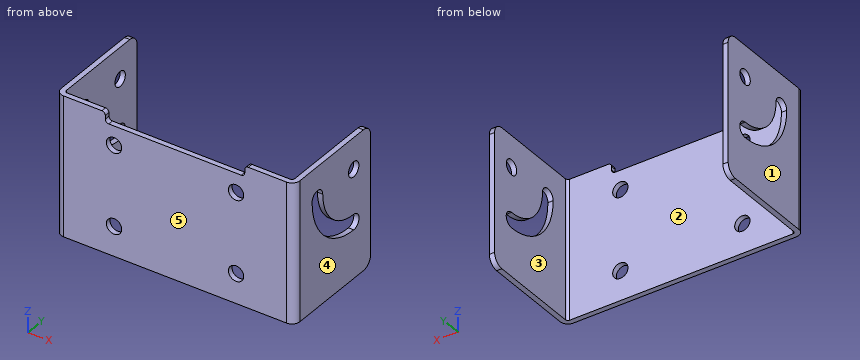
from build123d import *

# Parameters (mm, degrees)
SKETCH_1_W                         = 65.5
SKETCH_1_H                         = 40
SKETCH_1_R                         = 2.2
SM_BASE_FLANGE_1_DEPTH             = 1.5
SM_EDGE_FLANGE_1_STRIP_W           = 7.4732
SM_EDGE_FLANGE_1_STRIP_H           = 1.5
SM_EDGE_FLANGE_1_STRIP_CUT_DEPTH   = 40
SM_EDGE_FLANGE_1_STRIP_2_W         = 7.4732
SM_EDGE_FLANGE_1_STRIP_2_H         = 1.5
SM_EDGE_FLANGE_1_STRIP_CUT_2_DEPTH = 40
SM_EDGE_FLANGE_1_DEPTH             = 40
SM_EDGE_FLANGE_1_BEND_DEPTH        = 40
SKETCH_12_R                        = 2.15
CUT_EXTRUDE_1_DEPTH                = 78.409624725
SKETCH_13_W                        = 40
SKETCH_13_H                        = 3
CUT_EXTRUDE_2_DEPTH                = 50.729895435
FILLET_1_R                         = 1
FILLET_2_R                         = 3


# Sheet-metal steps are written as plain solids
with BuildPart() as part:
    # Sketch 1 → 基体-法兰1 (new body)
    with BuildSketch(Plane(origin=(0, 0, 0), x_dir=(1, 0, 0), z_dir=(0, 1, 0))):
        Rectangle(SKETCH_1_W, SKETCH_1_H)
        with Locations(Location((-17.5, 11.5, 0), (0, 0, 270))):
            Circle(SKETCH_1_R, mode=Mode.SUBTRACT)
        with Locations(Location((17.5, 11.5, 0), (0, 0, 270))):
            Circle(SKETCH_1_R, mode=Mode.SUBTRACT)
        with Locations(Location((17.5, -11.5, 0), (0, 0, 270))):
            Circle(SKETCH_1_R, mode=Mode.SUBTRACT)
        with Locations(Location((-17.5, -11.5, 0), (0, 0, 270))):
            Circle(SKETCH_1_R, mode=Mode.SUBTRACT)
    extrude(amount=-SM_BASE_FLANGE_1_DEPTH)

    # 边线-法兰1 strip (across the edge) → 边线-法兰1 strip cut (cut)
    with BuildSketch(Plane(origin=(-32.75, 0, -20), x_dir=(1, 0, 0), z_dir=(0, 0, 1))):
        with Locations((-3, -0.75)):
            Rectangle(SM_EDGE_FLANGE_1_STRIP_W, SM_EDGE_FLANGE_1_STRIP_H)
    extrude(amount=SM_EDGE_FLANGE_1_STRIP_CUT_DEPTH, mode=Mode.SUBTRACT)

    # 边线-法兰1 strip 2 (across the edge) → 边线-法兰1 strip cut 2 (cut)
    with BuildSketch(Plane(origin=(32.75, 0, 20), x_dir=(-1, 0, 0), z_dir=(0, 0, -1))):
        with Locations((-3, -0.75)):
            Rectangle(SM_EDGE_FLANGE_1_STRIP_2_W, SM_EDGE_FLANGE_1_STRIP_2_H)
    extrude(amount=SM_EDGE_FLANGE_1_STRIP_CUT_2_DEPTH, mode=Mode.SUBTRACT)

    # 边线-法兰1 section (across the edge) → 边线-法兰1 (add)
    with BuildSketch(Plane(origin=(-32.75, 0, -20), x_dir=(1, 0, 0), z_dir=(0, 0, 1))):
        with BuildLine():
            Line((-1.5, 0.7366), (-1.5, 30))
            Line((-1.5, 30), (0, 30))
            Line((0, 30), (0, 0.7366))
            ThreePointArc((0, 0.7366), (0.215745145, 0.215745145), (0.7366, 0))
            Line((0.7366, 0), (0.7366, -1.5))
            ThreePointArc((0.7366, -1.5), (-0.844915027, -0.844915027), (-1.5, 0.7366))
        make_face()
    extrude(amount=SM_EDGE_FLANGE_1_DEPTH)

    # 边线-法兰1 section 2 (across the edge) → 边线-法兰1 bend (add)
    with BuildSketch(Plane(origin=(32.75, 0, 20), x_dir=(-1, 0, 0), z_dir=(0, 0, -1))):
        with BuildLine():
            Line((-1.5, 0.7366), (-1.5, 30))
            Line((-1.5, 30), (0, 30))
            Line((0, 30), (0, 0.7366))
            ThreePointArc((0, 0.7366), (0.215745145, 0.215745145), (0.7366, 0))
            Line((0.7366, 0), (0.7366, -1.5))
            ThreePointArc((0.7366, -1.5), (-0.844915027, -0.844915027), (-1.5, 0.7366))
        make_face()
    extrude(amount=SM_EDGE_FLANGE_1_BEND_DEPTH)

    # 草图12 → 切除-拉伸1 (cut, through all)
    with BuildSketch(Plane.ZY.offset(34.25)):
        with Locations(Location((11, 23, 0), (0, 0, 270))):
            Circle(SKETCH_12_R)
        with BuildLine():
            ThreePointArc((-6.2, 23), (-1.162236636, 10.837763364), (11, 5.8))
            ThreePointArc((11, 5.8), (13.2, 8), (11, 10.2))
            ThreePointArc((11, 10.2), (1.949033201, 13.949033201), (-1.8, 23))
            ThreePointArc((-1.8, 23), (-4, 25.2), (-6.2, 23))
        make_face()
    extrude(amount=-CUT_EXTRUDE_1_DEPTH, mode=Mode.SUBTRACT)

    # 草图13 → 切除-拉伸2 (cut, through all)
    with BuildSketch(Plane(origin=(0, 0, 0), x_dir=(1, 0, 0), z_dir=(0, 1, 0))):
        with Locations((0, -18.5)):
            Rectangle(SKETCH_13_W, SKETCH_13_H)
    extrude(amount=-CUT_EXTRUDE_2_DEPTH, mode=Mode.SUBTRACT)

    # 圆角1
    fillet_1_edges = [part.edges().sort_by_distance(p)[0] for p in [
        (-20, -0.75, 20),
        (-20, -0.75, 17),
        (20, -0.75, 17),
        (20, -0.75, 20),
    ]]
    fillet(fillet_1_edges, radius=FILLET_1_R)

    # 圆角2
    fillet_2_edges = [part.edges().sort_by_distance(p)[0] for p in [
        (-33.5, 30, -20),
        (-33.5, 30, 20),
        (33.5, 30, 20),
        (33.5, 30, -20),
    ]]
    fillet(fillet_2_edges, radius=FILLET_2_R)


solid = part.part
Build history of the part. All positions in model axes, mm. Face numbers are marked on the shaded views. A direction names the side the tool comes from. Coordinates: 2 decimals unless noted, no trailing zeros. Write each loop counter-clockwise with the first axis right and the second up, starting at its lowest first coordinate (ties: lowest second). Pieces come first, ordered by that corner, then holes.
(1) Mould opens along X. For the marked faces 3, 4 and 5 say: pulls with the +X half, pulls with the -X half, needs draft (parallel to the pull), parting line crosses it, or undercut.
(2) Cut at B-B on z = -11.5. List the corners of the cut face in (x, y).
(3) Drill centre lines: line 1 (X direction, y = 12, z = 11); line 2 (X direction, y = -1.1, z = -11.5); line 3 (X direction, y = -0.85, z = 11.5). Where is each one in solid material? Low to high.
(4) 3-axis set-ups, long thin cutter, end or side, ignore diameter. For the marked faces 1 and 2: which of +Z, -Z, +X, -X, +Y, -Y reach the whole face in a straight line?
(5) Pin check, flat tips, straight feed: pin 1 Ø2.5 at (x, z) = (17.5, 11.5) entering from -Y; pin 2 Ø2 at (x, z) = (-3.5, -10) entering from +Y; pin 3 Ø1.1 at (y, z) = (-0.5, 18.5) entering from -X. Stop position of each tip, or through.
(6) Cut at D-D on y = 22. List the corners of the cut face in (x, z), and give its area (4 significant figures).
(7) Cut at C-C on y = 13. List the corners of the cut face in (x, z), and give its area (3 significant figures).
(8) Cut at A-A on x = -17.5. List the corners of the cut face in (y, z).
Working result:
1. face 3: undercut
1. face 4: pulls with the +X half
1. face 5: needs draft
2. outline: (-34.25, 0.74) arc R2.24 ccw to (-32.01, -1.5) - (-19.7, -1.5) - (-19.7, 0) - (-32.01, 0) arc R0.74 cw to (-32.75, 0.74) - (-32.75, 30) - (-34.25, 30) - close; (-15.3, -1.5) - (15.3, -1.5) - (15.3, 0) - (-15.3, 0) - close; (19.7, -1.5) - (32.01, -1.5) arc R2.24 ccw to (34.25, 0.74) - (34.25, 30) - (32.75, 30) - (32.75, 0.74) arc R0.74 cw to (32.01, 0) - (19.7, 0) - close
3. line 1: x = -34.25 to -32.75, 32.75 to 34.25
3. line 2: x = -33.29 to -19.7, -15.3 to 15.3, 19.7 to 33.29
3. line 3: x = -33.59 to -19.7, -15.3 to 15.3, 19.7 to 33.59
4. face 1: +Z, -Z, -X, +Y, -Y
4. face 2: +Z, -Z, +Y
5. pin 1: passes through
5. pin 2: stops at y = 0
5. pin 3: stops at x = -34.14
6. outline: (-34.25, -20) - (-32.75, -20) - (-32.75, -6.17) - (-34.25, -6.17) - close; (-34.25, -1.76) - (-32.75, -1.76) - (-32.75, 9.1) - (-34.25, 9.1) - close; (-34.25, 12.9) - (-32.75, 12.9) - (-32.75, 20) - (-34.25, 20) - close; (32.75, -20) - (34.25, -20) - (34.25, -6.17) - (32.75, -6.17) - close; (32.75, -1.76) - (34.25, -1.76) - (34.25, 9.1) - (32.75, 9.1) - close; (32.75, 12.9) - (34.25, 12.9) - (34.25, 20) - (32.75, 20) - close
6. area: 95.35 mm2
7. outline: (-34.25, -20) - (-32.75, -20) - (-32.75, -2.99) - (-34.25, -2.99) - close; (-34.25, 3.01) - (-32.75, 3.01) - (-32.75, 20) - (-34.25, 20) - close; (32.75, -20) - (34.25, -20) - (34.25, -2.99) - (32.75, -2.99) - close; (32.75, 3.01) - (34.25, 3.01) - (34.25, 20) - (32.75, 20) - close
7. area: 102 mm2
8. outline: (-1.5, -20) - (0, -20) - (0, -13.7) - (-1.5, -13.7) - close; (-1.5, -9.3) - (0, -9.3) - (0, 9.3) - (-1.5, 9.3) - close; (-1.5, 13.7) - (0, 13.7) - (0, 17) - (-1.5, 17) - close
